from build123d import *

# Parameters (mm, degrees)
SKETCH_1_R                   = 2.9
EXTRUDE_1_DEPTH              = 3.5
SKETCH_2_R                   = 2.5
EXTRUDE_2_DEPTH              = 10.5
CUT_EXTRUDE_1_DEPTH          = 3.5
HOLE_WIZARD_M3_1_D           = 2.5
HOLE_WIZARD_M3_1_DEPTH       = 8
HOLE_WIZARD_M3_1_CSINK_D     = 3.2
HOLE_WIZARD_M3_1_CSINK_ANGLE = 90
HOLE_WIZARD_M3_1_TIP         = 1.25


with BuildPart() as part:
    # 草图1 → 凸台-拉伸1 (new body)
    with BuildSketch(Plane(origin=(0, 0, 0), x_dir=(1, 0, 0), z_dir=(0, 1, 0))):
        with Locations(Location((0, 0, 0), (0, 0, 270))):
            Circle(SKETCH_1_R)
    extrude(amount=EXTRUDE_1_DEPTH)

    # 草图2 → 凸台-拉伸2 (add)
    with BuildSketch(Plane(origin=(0, 3.5, 0), x_dir=(1, 0, 0), z_dir=(0, 1, 0))):
        with Locations(Location((0, 0, 0), (0, 0, 90))):
            Circle(SKETCH_2_R)
    extrude(amount=EXTRUDE_2_DEPTH)

    # 草图3 → 切除-拉伸1 (cut)
    with BuildSketch(Plane.XZ):
        Polygon((0, 2.55), (0.366495157, 2.916495157), (-0.366495157, 2.916495157), align=None)
        Polygon((0.634159212, 2.469887061), (1.080283889, 2.733724459), (0.370321814, 2.916011738), align=None)
        Polygon((1.228471869, 2.234582034), (1.726194412, 2.3791838), (1.083870103, 2.732304577), align=None)
        Polygon((1.74559512, 1.85887), (2.263641791, 1.875150272), (1.729314848, 2.37691667), align=None)
        Polygon((2.15303621, 1.366358327), (2.658856231, 1.253294157), (2.26610038, 1.872178348), align=None)
        Polygon((2.425194117, 0.787993336), (2.887004956, 0.55268896), (2.660498492, 1.249804175), align=None)
        Polygon((2.544968157, 0.160115825), (2.933752541, -0.182643716), (2.887727699, 0.548900209), align=None)
        Polygon((2.504832489, -0.477822352), (2.796161665, -0.906500217), (2.933510354, -0.186493176), align=None)
        Polygon((2.307308984, -1.085737193), (2.482877668, -1.573397974), (2.794969765, -0.910168509), align=None)
        Polygon((1.964808769, -1.625431174), (2.013585336, -2.141433351), (2.480810946, -1.576654607), align=None)
        Polygon((1.498852393, -2.062993336), (1.417772031, -2.574914594), (2.010773652, -2.144073698), align=None)
        Polygon((0.938717609, -2.370930039), (0.732874896, -2.846604484), (1.414392054, -2.576772752), align=None)
        Polygon((0.319599746, -2.529892488), (0.001928536, -2.939431745), (0.729139002, -2.847563698), align=None)
        Polygon((-0.319599746, -2.529892488), (-0.729139002, -2.847563698), (-0.001928536, -2.939431745), align=None)
        Polygon((-0.938717609, -2.370930039), (-1.414392054, -2.576772752), (-0.732874896, -2.846604484), align=None)
        Polygon((-1.498852393, -2.062993336), (-2.010773652, -2.144073698), (-1.417772031, -2.574914594), align=None)
        Polygon((-1.964808769, -1.625431174), (-2.480810946, -1.576654607), (-2.013585336, -2.141433351), align=None)
        Polygon((-2.307308984, -1.085737193), (-2.794969765, -0.910168509), (-2.482877668, -1.573397974), align=None)
        Polygon((-2.504832489, -0.477822352), (-2.933510354, -0.186493176), (-2.796161665, -0.906500217), align=None)
        Polygon((-2.544968157, 0.160115825), (-2.887727699, 0.548900209), (-2.933752541, -0.182643716), align=None)
        Polygon((-2.425194117, 0.787993336), (-2.660498492, 1.249804175), (-2.887004956, 0.55268896), align=None)
        Polygon((-2.15303621, 1.366358327), (-2.26610038, 1.872178348), (-2.658856231, 1.253294157), align=None)
        Polygon((-1.74559512, 1.85887), (-1.729314848, 2.37691667), (-2.263641791, 1.875150272), align=None)
        Polygon((-1.228471869, 2.234582034), (-1.083870103, 2.732304577), (-1.726194412, 2.3791838), align=None)
        Polygon((-0.634159212, 2.469887061), (-0.370321814, 2.916011738), (-1.080283889, 2.733724459), align=None)
    extrude(amount=-CUT_EXTRUDE_1_DEPTH, mode=Mode.SUBTRACT)

    # M3 螺旋的螺纹孔钻头1
    with Locations(Plane(origin=(0, 0, 0), x_dir=(-1, 0, 0), z_dir=(0, -1, 0))):
        with Locations((0, 0)):
            CounterSinkHole(HOLE_WIZARD_M3_1_D / 2, HOLE_WIZARD_M3_1_CSINK_D / 2, depth=HOLE_WIZARD_M3_1_DEPTH, counter_sink_angle=HOLE_WIZARD_M3_1_CSINK_ANGLE)
            with Locations((0, 0, -(HOLE_WIZARD_M3_1_DEPTH + HOLE_WIZARD_M3_1_TIP / 2))):  # 90° drill point
                Cone(0, HOLE_WIZARD_M3_1_D / 2, HOLE_WIZARD_M3_1_TIP, mode=Mode.SUBTRACT)


solid = part.part
Could you check a few things on this model? Use its own coordinates, in mm. A direction names the side the tool comes from. Give positions to 0.01 mm unless a question says otherwise; leave off trailing zeros. Loops run counter-clockwise (first coordinate to the right, second up) from the corner with the lowest first, then second, coordinate; pieces in that order, holes last. Notation, with made-up numbers: (69.5, 2.25) -> (107.5, 2.25) arc R10 ccw to (107.5, 20.25) -> close; hole circle Ø3 at (1, 85.5). An arc over 180 degrees is marked (long way). Answer as CSV lines item,"result". Start each with the question number.
(1) I need wall thicknesses on probe 1 along Z at (x, y) = (0.7, 7.75); probe 2 along Z at (x, y) = (-0.6, 6); probe 3 along X at (y, z) = (9.25, 0.8). Which ranges of each line are inside material? Lowest first, please.
(2) If we section it at B-B on y = 13.25: Write out the boundary of the cut face in (x, z), then the cut area to 3 significant figures.
(3) We'd pull the mould along X, two halves only. Please class faces 3 (the cylindrical face through (2.44, 8.68, 0.54)), 4 (the conical face through (0.08, 8.89, 0.35)), 5 (the flat face through (-1.2, 0, -1.3)): released by +X, released by -X, zero draft, split by the parting line, or undercut.
(4) I'm going to push flat-ended pins straight in: pin 1 Ø3 at (x, y) = (-2, 10) entering from -Z; pin 2 Ø3 at (x, z) = (0, 0) entering from -Y; pin 3 Ø3 at (y, z) = (12.5, 1) entering from +X. Where does each tip first touch, or does it pass through?
(5) If we section it at A-A on y = 3.75: Write out the boundary of the cut face in (x, z).
(6) Which directions (+Z, -Z, +X, -X, +Y, -Y) give clear straight access to the entire face, cutting with the end or side of a thin tool? Please do faces 1 (the flat face through (0, 14, 0)), 2 (the cylindrical face through (-0.27, 4.23, 1.22)).
Computed:
1,probe 1,"z = -2.4 to -1.04, 1.04 to 2.4"
1,probe 2,"z = -2.43 to -1.1, 1.1 to 2.43"
1,probe 3,"x = -2.37 to 2.37"
2,outline,"circle Ø5 at (0, 0)"
2,area,"19.6 mm2"
3,face 3,"split by the parting line"
3,face 4,"undercut"
3,face 5,"zero draft"
4,pin 1,"stops at z = -2.45"
4,pin 2,"stops at y = 0.1"
4,pin 3,"stops at x = 2.5"
5,outline,"circle Ø5 at (0, 0); hole circle Ø2.5 at (0, 0)"
6,face 1,"+Z, -Z, +X, -X, +Y"
6,face 2,"-Y"
